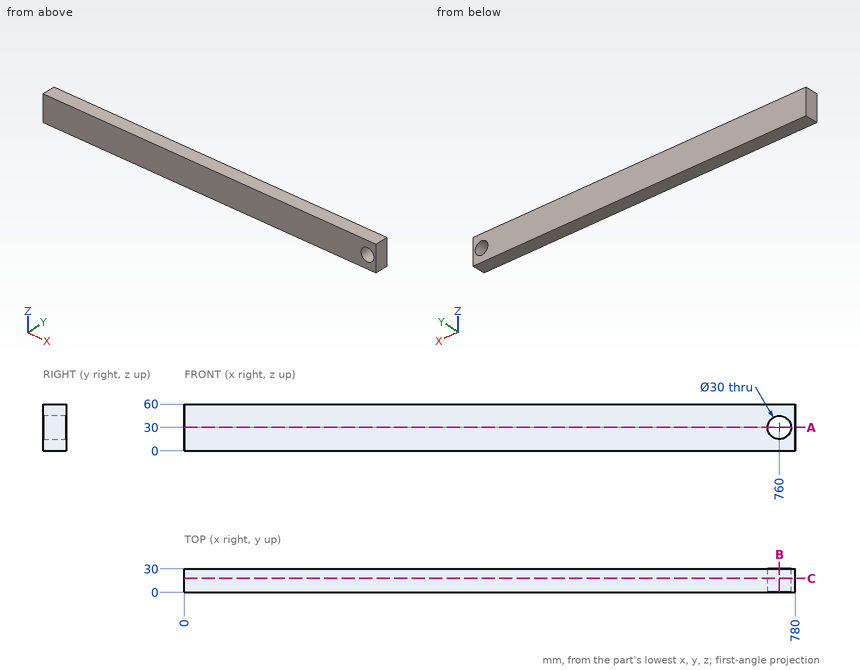
Answer from the drawing. Dimensions are ordinates in mm from the lowest x, y and z of the part. Coordinates: 2 decimals unless noted, no trailing zeros. Write each loop counter-clockwise with the first axis right and the second up, starting at its lowest first coordinate (ties: lowest second). Pieces come first, ordered by that corner, then holes. Notation, with made-up numbers: M 14.25,86.25 L 52.25,86.25 A21 cw 52.25,122.25 Z; hole C 27,67.5 d10. An arc over 180 degrees is marked long. Use one line per item in the form item = value. Start each with the question number.
1. The part is cut by section B-B (x = 760). Give the vertices of the cut face in (y, z), plus the area to 3 significant figures.
2. This flat-tipped pin is pushed along its axis until it touches: P1, Ø5, axis at x = 200, z = 21.5, coming from the -Y side. Where does it stop, or does it pass through?
3. The part is cut by section C-C (y = 18). Give the vertices of the cut face in (x, z).
4. Straight lines are drawn through the part: probe 1 along X at (y, z) = (7.75, 30); probe 2 along Z at (x, y) = (760, 7.5); probe 3 along X at (y, z) = (10.5, 39.5). For each, find the intervals that lie inside material, in ascending order. Write a range as from..to.
5. The part is cut by section A-A (z = 30). Give the vertices of the cut face in (x, y), plus the area to 3 significant figures.
Evaluation:
q1.outline = M 0,0 L 30,0 L 30,15 L 0,15 Z; M 0,45 L 30,45 L 30,60 L 0,60 Z
q1.area = 900 mm^2
q2.P1 = 0
q3.outline = M 0,0 L 780,0 L 780,60 L 0,60 Z; hole C 760,30 d30
q4.probe_1 = 0..745, 775..780
q4.probe_2 = 0..15, 45..60
q4.probe_3 = 0..748.39, 771.61..780
q5.outline = M 0,0 L 745,0 L 745,30 L 0,30 Z; M 775,0 L 780,0 L 780,30 L 775,30 Z
q5.area = 22,500 mm^2
